Geometry check sheet. Reference: the model listing, model coordinates, mm. A direction names the side the tool comes from. Give positions to 0.01 mm unless a question says otherwise; leave off trailing zeros. Loops run counter-clockwise (first coordinate to the right, second up) from the corner with the lowest first, then second, coordinate; pieces in that order, holes last. Notation, with made-up numbers: (15.5, -14) -> (26.5, -14) arc R31 cw to (26.5, 16) -> close; hole circle Ø7 at (-24, -32). An arc over 180 degrees is marked (long way). Answer as a JSON object with one key per item and string values.
from build123d import *

# Parameters (mm, degrees)
F1_DEPTH  = 19.05
F2_R      = 9.525
F3_DEPTH  = 19.05
F4_R      = 6.35
F5_DEPTH  = 19.05
F6_R      = 6.35
F7_DEPTH  = 19.05
F8_DEPTH  = 19.05
F9_R      = 4.7625
F10_DEPTH = 19.05
F11_R     = 3.175
F12_DEPTH = 19.05


with BuildPart() as f1:
    # F0 (on Top) → F1 (new body)
    with BuildSketch(Plane.XY):
        Polygon((434.815569, 321.845666), (-479.584431, 321.845666), (-479.584431, -287.754334), (-123.984431, -287.754334), (-123.984431, -84.554334), (180.815569, -84.554334), (180.815569, -287.754334), (434.815569, -287.754334), align=None)
    extrude(amount=F1_DEPTH)

    # F2 (on face) → F3 (cut)
    with BuildSketch(Plane.XY.offset(19.05)):
        with Locations((-149.384431, -59.154334)):
            Circle(F2_R)
        with Locations((-149.384431, -135.354334)):
            Circle(F2_R)
        with Locations((-149.384431, -211.554334)):
            Circle(F2_R)
        with Locations((206.215569, -211.554334)):
            Circle(F2_R)
        with Locations((206.215569, -135.354334)):
            Circle(F2_R)
        with Locations((206.215569, -59.154334)):
            Circle(F2_R)
    extrude(amount=-F3_DEPTH, mode=Mode.SUBTRACT)

    # F4 (on face) → F5 (cut)
    with BuildSketch(Plane.XY.offset(19.05)):
        with Locations((345.915569, -268.704334)):
            Circle(F4_R)
        with Locations((422.115569, -268.704334)):
            Circle(F4_R)
        with Locations((-314.484431, -268.704334)):
            Circle(F4_R)
        with Locations((-390.684431, -268.704334)):
            Circle(F4_R)
        with Locations((-466.884431, -268.704334)):
            Circle(F4_R)
    extrude(amount=-F5_DEPTH, mode=Mode.SUBTRACT)

    # F6 (on face) → F7 (cut)
    with BuildSketch(Plane.XY.offset(19.05)):
        with Locations((-466.884431, -135.354334)):
            Circle(F6_R)
        with Locations((-466.884431, -33.754334)):
            Circle(F6_R)
        with Locations((-466.884431, 169.445666)):
            Circle(F6_R)
        with Locations((-466.884431, 67.845666)):
            Circle(F6_R)
        with Locations((422.115569, -33.754334)):
            Circle(F6_R)
        with Locations((422.115569, 67.845666)):
            Circle(F6_R)
        with Locations((422.115569, 169.445666)):
            Circle(F6_R)
        with Locations((422.115569, 271.045666)):
            Circle(F6_R)
        with Locations((422.115569, -135.354334)):
            Circle(F6_R)
        with Locations((-466.884431, 271.045666)):
            Circle(F6_R)
        with Locations((-466.884431, 309.145666)):
            Circle(F6_R)
        with Locations((422.115569, 309.145666)):
            Circle(F6_R)
        with Locations((-289.084431, 309.145666)):
            Circle(F6_R)
        with Locations((-111.284431, 309.145666)):
            Circle(F6_R)
        with Locations((66.515569, 309.145666)):
            Circle(F6_R)
        with Locations((244.315569, 309.145666)):
            Circle(F6_R)
        with Locations((-149.384431, 271.045666)):
            Circle(F6_R)
        with Locations((104.615569, 283.745666)):
            Circle(F6_R)
        with Locations((-149.384431, 194.845666)):
            Circle(F6_R)
        with Locations((104.615569, 194.845666)):
            Circle(F6_R)
        with Locations((-352.584431, 17.045666)):
            Circle(F6_R)
        with Locations((-220.504431, 17.045666)):
            Circle(F6_R)
        with Locations((-88.424431, 17.045666)):
            Circle(F6_R)
        with Locations((43.655569, 17.045666)):
            Circle(F6_R)
        with Locations((175.735569, 17.045666)):
            Circle(F6_R)
        with Locations((307.815569, 17.045666)):
            Circle(F6_R)
        with Locations((-174.784431, 144.045666)):
            Circle(F6_R)
        with Locations((41.115569, 144.045666)):
            Circle(F6_R)
        with Locations((-174.784431, 42.445666)):
            Circle(F6_R)
        with Locations((41.115569, 42.445666)):
            Circle(F6_R)
    extrude(amount=-F7_DEPTH, mode=Mode.SUBTRACT)

    # F4 (on face) → F8 (cut)
    with BuildSketch(Plane.XY.offset(19.05)):
        with Locations((-466.884431, -268.704334)):
            Circle(F4_R)
        with Locations((-390.684431, -268.704334)):
            Circle(F4_R)
        with Locations((-314.484431, -268.704334)):
            Circle(F4_R)
        with Locations((345.915569, -268.704334)):
            Circle(F4_R)
        with Locations((422.115569, -268.704334)):
            Circle(F4_R)
    extrude(amount=-F8_DEPTH, mode=Mode.SUBTRACT)

    # F9 (on face) → F10 (cut)
    with BuildSketch(Plane.XY.offset(19.05)):
        with Locations((-403.384431, 290.095666)):
            Circle(F9_R)
        with Locations((-365.284431, 290.095666)):
            Circle(F9_R)
        with Locations((320.515569, 290.095666)):
            Circle(F9_R)
        with Locations((358.615569, 290.095666)):
            Circle(F9_R)
        with Locations((-403.384431, 86.895666)):
            Circle(F9_R)
        with Locations((-365.284431, 86.895666)):
            Circle(F9_R)
        with Locations((320.515569, 86.895666)):
            Circle(F9_R)
        with Locations((358.615569, 86.895666)):
            Circle(F9_R)
    extrude(amount=-F10_DEPTH, mode=Mode.SUBTRACT)

    # F11 (on face) → F12 (cut)
    with BuildSketch(Plane.XY.offset(19.05)):
        with Locations((-397.034431, 74.195666)):
            Circle(F11_R)
        with Locations((-397.034431, 55.145666)):
            Circle(F11_R)
        with Locations((352.265569, 74.195666)):
            Circle(F11_R)
        with Locations((352.265569, 55.145666)):
            Circle(F11_R)
    extrude(amount=-F12_DEPTH, mode=Mode.SUBTRACT)


solid = f1.part
1) Material ranges on line 1 along Y through (x, z) = (358, 14); line 2 along X through (y, z) = (-136, 7); line 3 along X through (y, z) = (55.5, 8.5), recorded low to high. Write a range as from..to.
Geometry check:
{"line 1": "y = -287.75..82.17, 91.62..285.37, 294.82..321.85", "line 2": "x = -479.58..-473.2, -460.57..-158.89, -139.88..-123.98, 180.82..196.71, 215.72..415.8, 428.43..434.82", "line 3": "x = -479.58..-400.19, -393.88..349.11, 355.42..434.82"}
2) Draft check along X on faces 1 (the face through (-479.584, 21, 9)), 2 (the face through (434.816, 13, 9)), 3 (the face through (-144.989, -220.005, 9.658)). Enter one of: pulls with the +X half, pulls with the -X half, needs draft (parallel to the pull), parting line crosses it, or undercut.
Geometry check:
{"face 1": "pulls with the -X half", "face 2": "pulls with the +X half", "face 3": "undercut"}
3) Section check B-B on x = 123.5. Record the cut outline in (y, z), plus the area to 3 significant figures.
Geometry check:
{"outline": "(-84.55, 0) -> (321.85, 0) -> (321.85, 19.05) -> (-84.55, 19.05) -> close", "area": "7,740 mm2"}
4) Depth check by flat-ended pin: P1, Ø20.5, axis at x = 175.74, y = 17.05, coming from the +Z side; P2, Ø17, axis at x = -149.38, y = -59.15, coming from the -Z side; P3, Ø1.5, axis at x = 5.5, z = 17, coming from the -Y side. Enter the tip coordinate at first touch or a pass-through.
Geometry check:
{"P1": "stops at z = 19.05", "P2": "passes through", "P3": "stops at y = -84.55"}
5) Section check A-A on y = -171.5. Record the cut outline in (x, z), plus the area to 3 significant figures.
Geometry check:
{"outline": "(-479.58, 0) -> (-123.98, 0) -> (-123.98, 19.05) -> (-479.58, 19.05) -> close; (180.82, 0) -> (434.82, 0) -> (434.82, 19.05) -> (180.82, 19.05) -> close", "area": "11,600 mm2"}
6) Section check C-C on z = 15.5. Count the separate pieces of the cut face and the enclosed holes in it, plus the area to 3 significant figures.
Geometry check:
{"separate pieces": "1", "enclosed holes": "53", "area": "489,000 mm2"}
7) Tool access check on faces 4 (the face through (26, -84.554, 9)), 5 (the face through (-304, -287.754, 9)). Record the directions out of +Z, -Z, +X, -X, +Y, -Y that give a thin tool (end or side, any length) a straight path to the whole face; none if there is none.
Geometry check:
{"face 4": "+Z, -Z, -Y", "face 5": "+Z, -Z, +X, -X, -Y"}
